```python
from build123d import *

# Parameters (mm, degrees)
F0_W     = 101.6
F0_H     = 63.5
F1_DEPTH = 12.7
F2_R     = 6.35
F3_DEPTH = 25.4
F4_W     = 19.05
F4_H     = 38.1
F6_W     = 12.7
F6_H     = 12.7


with BuildPart() as f1:
    # F0 (on Top) → F1 (new body)
    with BuildSketch(Plane.XY):
        Rectangle(F0_W, F0_H)
    extrude(amount=F1_DEPTH)

    # F2 (on face) → F3 (cut)
    with BuildSketch(Plane.XY.offset(12.7)):
        with Locations((-38.1, 19.05)):
            Circle(F2_R)
        with Locations((-38.1, -19.05)):
            Circle(F2_R)
        with Locations((38.1, -19.05)):
            Circle(F2_R)
        with Locations((38.1, 19.05)):
            Circle(F2_R)
    extrude(amount=-F3_DEPTH, mode=Mode.SUBTRACT)

    # F4 (on Front) → F5 (revolve)
    with BuildSketch(Plane.XZ):
        with Locations((-9.525, 31.75)):
            Rectangle(F4_W, F4_H)
    revolve(axis=Axis((0, 0, 31.75), (0, 0, 1)))

    # F6 (on Front) → F7 (revolve, cut)
    with BuildSketch(Plane.XZ):
        with Locations((-19.05, 33.404847)):
            Rectangle(F6_W, F6_H)
    revolve(axis=Axis((0, 0, 21.012729), (0, 0, -1)), mode=Mode.SUBTRACT)


solid = f1.part
```
Work out the finished part from the listing and answer in its coordinate system (mm). A direction names the side the tool comes from. Coordinates: 2 decimals unless noted, no trailing zeros. Write each loop counter-clockwise with the first axis right and the second up, starting at its lowest first coordinate (ties: lowest second). Pieces come first, ordered by that corner, then holes.
Q1. Find the intervals of material crossed by line 1 (Y direction, x = 38.1, z = 8.75); line 2 (X direction, y = 19, z = 8); line 3 (X direction, y = 15, z = 7.5), in increasing order.
Q2. A cutting plane is placed at C-C, the plane z = 4. Give the vertices of the cut face in (x, y), then the cut area to 3 significant figures.
Q3. Which of the six approach directions +Z, -Z, +X, -X, +Y, -Y give full straight-line access (tool end or side, diameter ignored) to faces 4 (the face through (15.12, 11.59, 19.98)), 5 (the face through (-32.043, 20.957, 6.439)), 6 (the face through (1.653, 12.592, 33.494))?
Q4. A cutting plane is placed at D-D, the plane x = -18. Give the vertices of the cut face in (y, z), then the cut area to 3 significant figures.
Q5. A cutting plane is placed at A-A, the plane x = -38.1. Give the vertices of the cut face in (y, z), then the cut area to 3 significant figures.
Q6. A cutting plane is placed at B-B, the plane y = 14.5. Give the vertices of the cut face in (x, z), then the cut area to 3 significant figures.
Q7. Determine the mould class of faces 1 (the face through (15.12, 11.59, 45.35)), 2 (the face through (-12.4, -4, 39.755)), 3 (the face through (-32.234, -21.482, 6.439)) for opening direction X: released by +X, released by -X, zero draft, split by the parting line, or undercut.
Q8. Each of these flat-tipped pins is pushed along its axis until it touches: pin 1 Ø10 at (x, z) = (-13, 40.5) entering from -Y; pin 2 Ø6 at (y, z) = (22, 29.5) entering from -X; pin 3 Ø12 at (x, z) = (-14, 31.5) entering from -Y; pin 4 Ø8 at (y, z) = (-18.5, 45) entering from -X. Where does it stop, or does it pass through?
Findings below:
1. line 1: y = -31.75 to -25.4, -12.7 to 12.7, 25.4 to 31.75
1. line 2: x = -50.8 to -44.45, -31.75 to 31.75, 44.45 to 50.8
1. line 3: x = -50.8 to -42.99, -33.21 to 33.21, 42.99 to 50.8
2. outline: (-50.8, -31.75) - (50.8, -31.75) - (50.8, 31.75) - (-50.8, 31.75) - close; hole circle Ø12.7 at (-38.1, -19.05); hole circle Ø12.7 at (-38.1, 19.05); hole circle Ø12.7 at (38.1, -19.05); hole circle Ø12.7 at (38.1, 19.05)
2. area: 5,940 mm2
3. face 4: +Z
3. face 5: +Z, -Z
3. face 6: none
4. outline: (-31.75, 0) - (31.75, 0) - (31.75, 12.7) - (6.24, 12.7) - (6.24, 27.05) - (-6.24, 27.05) - (-6.24, 12.7) - (-31.75, 12.7) - close; (-6.24, 39.75) - (6.24, 39.75) - (6.24, 50.8) - (-6.24, 50.8) - close
4. area: 1,120 mm2
5. outline: (-31.75, 0) - (-25.4, 0) - (-25.4, 12.7) - (-31.75, 12.7) - close; (-12.7, 0) - (12.7, 0) - (12.7, 12.7) - (-12.7, 12.7) - close; (25.4, 0) - (31.75, 0) - (31.75, 12.7) - (25.4, 12.7) - close
5. area: 484 mm2
6. outline: (-50.8, 0) - (-42.53, 0) - (-42.53, 12.7) - (-50.8, 12.7) - close; (-33.67, 0) - (33.67, 0) - (33.67, 12.7) - (12.36, 12.7) - (12.36, 27.05) - (-12.36, 27.05) - (-12.36, 12.7) - (-33.67, 12.7) - close; (-12.36, 39.75) - (12.36, 39.75) - (12.36, 50.8) - (-12.36, 50.8) - close; (42.53, 0) - (50.8, 0) - (50.8, 12.7) - (42.53, 12.7) - close
6. area: 1,690 mm2
7. face 1: split by the parting line
7. face 2: zero draft
7. face 3: undercut
8. pin 1: stops at y = -17.29
8. pin 2: passes through
8. pin 3: stops at y = -16.23
8. pin 4: stops at x = -12.36
